```python
from build123d import *

# Parameters (mm, degrees)
F0_W      = 100
F0_H      = 45
F1_DEPTH  = 100
F2_W      = 65
F2_H      = 20
F3_DEPTH  = 100.001
F6_DEPTH  = 40
F7_W      = 10
F7_H      = 30
F8_DEPTH  = 45
F10_DEPTH = 100.001
F13_DEPTH = 85


with BuildPart() as f1:
    # F0 (on Top) → F1 (new body)
    with BuildSketch(Plane.XY):
        with Locations((50, 22.5)):
            Rectangle(F0_W, F0_H)
    extrude(amount=F1_DEPTH)

    # F2 (on face) → F3 (cut, through all)
    with BuildSketch(Plane.XY.offset(100)):
        with Locations((67.5, 10)):
            Rectangle(F2_W, F2_H)
    extrude(amount=-F3_DEPTH, mode=Mode.SUBTRACT)

    # F5 (on face) → F6 (cut, through all)
    with BuildSketch(Plane.XY.offset(100)):
        Polygon((35, 0), (35, 20), (35, 45), (15, 45), (0, 20), (0, 0), align=None)
    extrude(amount=-F6_DEPTH, mode=Mode.SUBTRACT)

    # F7 (on face) → F8 (cut)
    with BuildSketch(Plane.YZ.offset(100)):
        with Locations((25, 45)):
            Rectangle(F7_W, F7_H)
    extrude(amount=-F8_DEPTH, mode=Mode.SUBTRACT)

    # F9 (on face) → F10 (cut, through all)
    with BuildSketch(Plane.XY.offset(100)):
        Polygon((100, 20), (100, 45), (80, 20), align=None)
    extrude(amount=-F10_DEPTH, mode=Mode.SUBTRACT)

    # F12 (on face) → F13 (cut, through all)
    with BuildSketch(Plane.XY.offset(100)):
        Polygon((50, 45), (35, 45), (35, 26.397135), align=None)
    extrude(amount=-F13_DEPTH, mode=Mode.SUBTRACT)


solid = f1.part
```
Build history of the part. All positions in model axes, mm. A direction names the side the tool comes from. Give positions to 0.01 mm unless a question says otherwise; leave off trailing zeros. Loops run counter-clockwise (first coordinate to the right, second up) from the corner with the lowest first, then second, coordinate; pieces in that order, holes last. Notation, with made-up numbers: (28.25, -20) -> (86.25, -20) arc R29 cw to (86.25, 18) -> close; hole circle Ø7 at (-38, 64.5). An arc over 180 degrees is marked (long way). One line per question, with ' | ' between items. Start each with the question number.
1) 3-axis set-ups, long thin cutter, end or side, ignore diameter. For faces 1 (the flat face through (52, 20, 51)), 2 (the flat face through (72, 30, 45)), 3 (the flat face through (41, 38, 15)), 4 (the flat face through (35, 23, 80)): which of +Z, -Z, +X, -X, +Y, -Y reach the whole face in a straight line?
2) Cut at B-B (z = 42). Give the cut face in (x, y).
3) Probe L1, parallel to Y at x = 56, z = 48.5; L2, parallel to Z at x = 16, y = 33; L3, parallel to X at y = 12.5, z = 59. List the from-to ranges inside material, lowest first.
4) Pin check, flat tips, straight feed: pin 1 (4 mm diameter, centred on x = 21.5, y = 27.5, fed in from +Z); pin 2 (12 mm diameter, centred on x = 86, y = 34, fed in from -Z); pin 3 (9 mm diameter, centred on x = 71.5, z = 46, fed in from -Y); pin 4 (2 mm diameter, centred on y = 38, z = 78.5, fed in from +X). Stop position of each tip, or through.
5) Cut at D-D (x = 59). Give the cut face in (y, z), plus the area to 3 significant figures.
6) Cut at A-A (z = 84). Give the cut face in (x, y), plus the area to 3 significant figures.
7) Two-plate mould, pull along X, no slides. Class faces 5 (the flat face through (35, 36, 38)), 6 (the flat face through (60, 45, 49)), 7 (the flat face through (7.6, 32.67, 80.28)), 8 (the flat face through (35, 10, 30)): released by +X, released by -X, zero draft, split by the parting line, or undercut.
8) Cut at C-C (y = 36.5). Give the cut face in (x, z), plus the area to 3 significant figures.
Return value:
1) face 1: +Z, -Z, +X, -Y | face 2: +X, -Y | face 3: +Z, +Y | face 4: +Z, +Y, -Y
2) outline: (0, 0) -> (35, 0) -> (35, 20) -> (55, 20) -> (55, 30) -> (88, 30) -> (100, 45) -> (50, 45) -> (35, 26.4) -> (35, 45) -> (0, 45) -> close
3) L1: 30 to 45 | L2: 0 to 60 | L3: 0 to 35
4) pin 1: z = 60 | pin 2: z = 0 | pin 3: y = 30 | pin 4: x = 95.2
5) outline: (20, 0) -> (45, 0) -> (45, 100) -> (20, 100) -> (20, 60) -> (30, 60) -> (30, 30) -> (20, 30) -> close | area: 2,200 mm^2
6) outline: (0, 20) -> (15, 45) -> (0, 45) -> close; (35, 20) -> (80, 20) -> (100, 45) -> (50, 45) -> (35, 26.4) -> close | area: 1,420 mm^2
7) face 5: undercut | face 6: zero draft | face 7: undercut | face 8: released by +X
8) outline: (0, 0) -> (93.2, 0) -> (93.2, 100) -> (43.15, 100) -> (43.15, 15) -> (35, 15) -> (35, 60) -> (9.9, 60) -> (9.9, 100) -> (0, 100) -> close | area: 7,620 mm^2
